Input: part model. Units: mm. Frame: model coordinates. A direction names the side the tool comes from. Round coordinates to 2 decimals unless told otherwise and drop trailing zeros. Loops run counter-clockwise (first coordinate to the right, second up) from the corner with the lowest first, then second, coordinate; pieces in that order, holes last.
1) First-contact query: pin 1 (1 mm diameter, centred on y = 39.5, z = 2, fed in from +X). Flat tip, straight axial feed; report the tip coordinate or a pass-through.
2) Section A-A, the plane z = 1.8. Return loops of the section in (x, y).
3) Ray query, line 1 along Z through (x, y) = (-47.5, 45.5); line 2 along Y through (x, z) = (-46.5, 0.85); line 3 along Y through (x, z) = (-43.5, 2). Return the intervals inside material, ascending.
4) Access query for faces 1 (the face through (-47.786, 43.659, 1.74)), 2 (the face through (-43, 44, 3)). Directions: +Z, -Z, +X, -X, +Y, -Y. A direction counts if a zero-diameter tool reaches every point of the face in a straight line with its end or side. Return the directions, or none.
5) Section B-B, the plane z = 0.5. Return loops of the section in (x, y).
from build123d import *

# Parameters (mm, degrees)
F0_R     = 4.95
F1_DEPTH = 3
F2_R     = 6
F2_R_2   = 4.95
F3_DEPTH = 1
F4_SIZE  = 0.5


with BuildPart() as f1:
    # F0 (on Top) → F1 (new body)
    with BuildSketch(Plane.XY):
        with Locations((-42.84095, 43.441828)):
            Circle(F0_R)
    extrude(amount=F1_DEPTH)

    # F2 (on face) → F3 (join)
    with BuildSketch(Plane(origin=(0, 0, 0), x_dir=(1, 0, 0), z_dir=(0, 0, -1))):
        with Locations((-42.84095, -43.441828)):
            Circle(F2_R)
        with Locations((-42.84095, -43.441828)):
            Circle(F2_R_2, mode=Mode.SUBTRACT)
    extrude(amount=-F3_DEPTH)

    # F4
    f4_edges = [f1.edges().sort_by_distance(p)[0] for p in [
        (-47.79095, 43.441828, 3),
    ]]
    chamfer(f4_edges, length=F4_SIZE)


solid = f1.part
Final values:
1. pin 1: stops at x = -39.28
2. outline: circle Ø9.9 at (-42.84, 43.44)
3. line 1: z = 0 to 1
3. line 2: y = 38.69 to 48.2
3. line 3: y = 38.54 to 48.35
4. face 1: +Z
4. face 2: +Z, +X, -X, +Y, -Y
5. outline: circle Ø12 at (-42.84, 43.44)
